Read the model definition and answer for the solid it produces. Units are mm, in the model's axes. Face numbers are marked on the shaded views. Coordinates: 2 decimals unless noted, no trailing zeros. Order: outer loops, then holes, each group sorted by start corner. A loop starts at its lowest first (then second) coordinate and runs counter-clockwise, first axis right, second up. Notation, with made-up numbers: (-31.5, 18.5) -> (27.5, 18.5) arc R18 cw to (27.5, 30.5) -> close; hole circle Ø10 at (28, 9). An arc over 180 degrees is marked (long way). Answer as a JSON object with one key per item and string values. Group by question number.
1) Section D-D on y = -1.85 is taken. Determine the outline of the cut face in (x, z), and give its area (3 significant figures).
2) Consider L1, parallel to Y at x = 0, z = 9.95; L2, parallel to X at y = -0.5, z = 10; L3, parallel to X at y = 0.2, z = 10.25. Determine where each line is inside the solid, lowest interval first.
3) Given pin 1 (1.5 mm diameter, centred on y = 0.5, z = 6.5, fed in from +X); pin 2 (1 mm diameter, centred on y = 0.5, z = 9.5, fed in from +X), each flat-ended and moving along its own axis, determine where each tip first touches the part or whether it passes through.
4) Section C-C on z = 10.25 is taken. Determine the outline of the cut face in (x, y).
5) Section A-A on x = 0 is taken. Determine the outline of the cut face in (y, z).
6) Determine the mould class of the marked faces 1, 2 and 3 for opening direction Y: released by +Y, released by -Y, zero draft, split by the parting line, or undercut.
7) Section B-B on y = 0 is taken. Determine the outline of the cut face in (x, z).
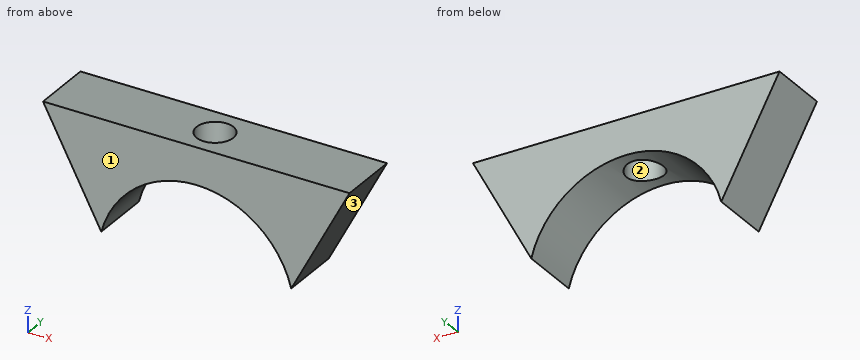
from build123d import *

# Parameters (mm, degrees)
F1_DEPTH = 2.5
F2_R     = 1.5
F3_DEPTH = 11.001


# Not quite as in the source:
# - a feature names something its author has since deleted; it is built from what else it names


with BuildPart() as f1:
    # F0 (on Front) → F1 (new body, symmetric)
    with BuildSketch(Plane.XZ):
        with BuildLine():
            Line((12.5, 11), (-12.5, 11))
            Line((-12.5, 11), (-7.7459666924, 2))
            ThreePointArc((-7.7459666924, 2), (0, 8), (7.7459666924, 2))
            Line((7.7459666924, 2), (12.5, 11))
        make_face()
    extrude(amount=F1_DEPTH, both=True)

    # F2 (on Top) → F3 (cut, through all)
    with BuildSketch(Plane.XY):
        Circle(F2_R)
    extrude(amount=F3_DEPTH, mode=Mode.SUBTRACT)


solid = f1.part
Worked answers:
{
 "1": {"outline": "(-12.5, 11) -> (-7.75, 2) arc R8 cw to (7.75, 2) -> (12.5, 11) -> close", "area": "113 mm²"},
 "2": {"L1": "y = -2.5 to -1.5, 1.5 to 2.5", "L2": "x = -11.97 to -1.41, 1.41 to 11.97", "L3": "x = -12.1 to -1.49, 1.49 to 12.1"},
 "3": {"pin 1": "stops at x = 10.52", "pin 2": "stops at x = 11.97"},
 "4": {"outline": "(-12.1, -2.5) -> (12.1, -2.5) -> (12.1, 2.5) -> (-12.1, 2.5) -> close; hole circle Ø3 at (0, 0)"},
 "5": {"outline": "(-2.5, 8) -> (-1.5, 8) -> (-1.5, 11) -> (-2.5, 11) -> close; (1.5, 8) -> (2.5, 8) -> (2.5, 11) -> (1.5, 11) -> close"},
 "6": {"face 1": "released by -Y", "face 2": "undercut", "face 3": "zero draft"},
 "7": {"outline": "(-12.5, 11) -> (-7.75, 2) arc R8 cw to (-1.5, 7.86) -> (-1.5, 11) -> close; (1.5, 7.86) arc R8 cw to (7.75, 2) -> (12.5, 11) -> (1.5, 11) -> close"}
}
